Could you check a few things on this model? Use its own coordinates, in mm. A direction names the side the tool comes from. Give positions to 0.01 mm unless a question says otherwise; leave off trailing zeros. Loops run counter-clockwise (first coordinate to the right, second up) from the corner with the lowest first, then second, coordinate; pieces in that order, holes last. Notation, with made-up numbers: (31, 23) - (59, 23) arc R12 ccw to (59, 30) - close; hole circle Ø10 at (44.25, 27). An arc over 180 degrees is marked (long way). Use CSV: the item, a comma, the result in double quotes.
from build123d import *

# Parameters (mm, degrees)
F1_DEPTH = 25.4
F2_DEPTH = 25.4
F3_R     = 5.08


with BuildPart() as f1:
    # F0 (on Front) → F1 (new body)
    with BuildSketch(Plane.XZ):
        with BuildLine():
            Line((-5.174372, -8.435566), (-43.773927, 20.35916))
            ThreePointArc((-43.773927, 20.35916), (-77.531681, 17.329487), (-78.223706, -16.556881))
            Line((-78.223706, -16.556881), (-5.174372, -101.541841))
            Line((-5.174372, -101.541841), (67.874961, -16.556881))
            ThreePointArc((67.874961, -16.556881), (67.182936, 17.329487), (33.425183, 20.35916))
            Line((33.425183, 20.35916), (-5.174372, -8.435566))
        make_face()
    extrude(amount=F1_DEPTH)

    # F0 (on Front) → F2 (join)
    with BuildSketch(Plane.XZ):
        with BuildLine():
            Line((-5.174372, -8.435566), (-43.773927, 20.35916))
            ThreePointArc((-43.773927, 20.35916), (-77.531681, 17.329487), (-78.223706, -16.556881))
            Line((-78.223706, -16.556881), (-5.174372, -101.541841))
            Line((-5.174372, -101.541841), (67.874961, -16.556881))
            ThreePointArc((67.874961, -16.556881), (67.182936, 17.329487), (33.425183, 20.35916))
            Line((33.425183, 20.35916), (-5.174372, -8.435566))
        make_face()
    extrude(amount=F2_DEPTH)

    # F3
    f3_edges = [f1.edges().sort_by_distance(p)[0] for p in [
        (-5.174372, -12.7, -8.435566),
    ]]
    fillet(f3_edges, radius=F3_R)


solid = f1.part
1) Suppose I cut it at A-A (y = -7.25). Please give me the cut outline in (x, z).
Answer below:
outline,"(-78.22, -16.56) - (-5.17, -101.54) - (67.87, -16.56) arc R25.4 ccw to (33.43, 20.36) - (-2.14, -6.17) arc R5.08 cw to (-8.21, -6.17) - (-43.77, 20.36) arc R25.4 ccw to start"
2) I need wall thicknesses on line 1 along X through (y, z) = (-15.25, 11); line 2 along Z through (x, y) = (-4, -7.25); line 3 along Z through (x, y) = (-23, -4.75). Which ranges of each line are inside material? Lowest first, please.
Answer below:
line 1,"x = -81.86 to -31.23, 20.88 to 71.51"
line 2,"z = -100.18 to -7.04"
line 3,"z = -80.8 to 4.86"
3) Suppose I cut it at B-B (z = -4). Please give me the cut outline in (x, y).
Answer below:
outline,"(-84.04, -25.4) - (-11.12, -25.4) - (-11.12, 0) - (-84.04, 0) - close; (0.77, -25.4) - (73.7, -25.4) - (73.7, 0) - (0.77, 0) - close"
4) Which directions (+Z, -Z, +X, -X, +Y, -Y) give clear straight access to the entire face, cutting with the end or side of a thin tool? Please do faces 4 (the flat face through (15.89, -12.52, 7.28)), 5 (the flat face through (-42.21, -12.522, -58.454)).
Answer below:
face 4,"+Z, +Y, -Y"
face 5,"-Z, -X, +Y, -Y"
5) We'd pull the mould along X, two halves only. Please class faces 1 (the flat face through (30.84, -12.52, -59.64)), 2 (the flat face through (-6, 0, -23)), 3 (the flat face through (-25.744, -12.522, 6.909)): +X half, -X half, draft (parallel to the pull), parting line (faces both ways), or undercut.
Answer below:
face 1,"+X half"
face 2,"draft"
face 3,"undercut"
6) Suppose I cut it at C-C (x = 38). Please give me the cut outline in (y, z).
Answer below:
outline,"(-25.4, -51.31) - (0, -51.31) - (0, 23.08) - (-25.4, 23.08) - close"
7) Suppose I cut it at D-D (z = -33). Please give me the cut outline in (x, y), plus the area to 3 significant figures.
Answer below:
outline,"(-64.09, -25.4) - (53.74, -25.4) - (53.74, 0) - (-64.09, 0) - close"
area,"2,990 mm2"
8) I'm going to push flat-ended pins straight in: P1, Ø1, axis at x = 44.5, y = -10, coming from the -Z side; P2, Ø12, axis at y = -20.5, z = -62.5, coming from the +X side; P3, Ø2, axis at x = -9.5, y = -19.5, coming from the -Z side. Where does each tip first touch, or does it pass through?
Answer below:
P1,"stops at z = -44.33"
P2,"stops at x = 33.54"
P3,"stops at z = -97.67"
